CAD build for the part. Positions are in the model's coordinates, mm. A direction names the side the tool comes from. Coordinates: 2 decimals unless noted, no trailing zeros. Write each loop counter-clockwise with the first axis right and the second up, starting at its lowest first coordinate (ties: lowest second). Pieces come first, ordered by that corner, then holes.
```python
from build123d import *

# Parameters (mm, degrees)
BOX010_W               = 4
BOX010_H               = 10
BOX010_DEPTH           = 7
BOX010_PLACEMENT_ANGLE = 95
BOX009_W               = 4
BOX009_H               = 10
BOX009_DEPTH           = 7
BOX009_PLACEMENT_ANGLE = 45
BOX011_W               = 3.5
BOX011_H               = 10
BOX011_DEPTH           = 6.9
BOX008_W               = 3.5
BOX008_H               = 10
BOX008_DEPTH           = 6.9
CUT007_PLACEMENT_ANGLE = 180
BOX006_W               = 4
BOX006_H               = 10
BOX006_DEPTH           = 7
BOX006_PLACEMENT_ANGLE = 95
BOX005_W               = 4
BOX005_H               = 10
BOX005_DEPTH           = 7
BOX005_PLACEMENT_ANGLE = 45
BOX007_W               = 3.5
BOX007_H               = 10
BOX007_DEPTH           = 6.9
BOX004_W               = 3.5
BOX004_H               = 10
BOX004_DEPTH           = 6.9
BOX003_W               = 34
BOX003_H               = 34
BOX003_DEPTH           = 10
SKETCH002_W            = 40
SKETCH002_H            = 90
PAD001_DEPTH           = 2


with BuildPart() as cube010:
    # Box010 → Box010 (new body)
    with BuildSketch(Plane.XY):
        with Locations((2, 5)):
            Rectangle(BOX010_W, BOX010_H)
    extrude(amount=BOX010_DEPTH)


with BuildPart() as cube010_1:
    # Box010 placement: moved
    add(cube010.part.moved(Location((18.35, -13, 15.9))).rotate(Axis((18.35, -13, 15.9), (0, 1, 0)), BOX010_PLACEMENT_ANGLE))


with BuildPart() as fusion003:
    # Box009 → Box009 (new body)
    with BuildSketch(Plane.XY):
        with Locations((2, 5)):
            Rectangle(BOX009_W, BOX009_H)
    extrude(amount=BOX009_DEPTH)


with BuildPart() as fusion003_1:
    # Box009 placement: moved
    add(fusion003.part.moved(Location((16, -13, 7))).rotate(Axis((16, -13, 7), (0, 1, 0)), BOX009_PLACEMENT_ANGLE))

    # Fusion003: union Cube010
    add(cube010_1.part)


with BuildPart() as fusion004:
    # Box011 → Box011 (new body)
    with BuildSketch(Plane(origin=(18, -13, 12), x_dir=(1, 0, 0), z_dir=(0, 0, 1))):
        with Locations((1.75, 5)):
            Rectangle(BOX011_W, BOX011_H)
    extrude(amount=BOX011_DEPTH)

    # Fusion004: union Fusion003
    add(fusion003_1.part)


with BuildPart() as obj1:
    # Box008 → Box008 (new body)
    with BuildSketch(Plane(origin=(16.5, -13, 9.1), x_dir=(1, 0, 0), z_dir=(0, 0, 1))):
        with Locations((1.75, 5)):
            Rectangle(BOX008_W, BOX008_H)
    extrude(amount=BOX008_DEPTH)

    # Cut007: cut Fusion004
    add(fusion004.part, mode=Mode.SUBTRACT)


with BuildPart() as obj1_1:
    # Cut007 placement: moved
    add(obj1.part.moved(Location((0, -16, 0))).rotate(Axis((0, -16, 0), (0, 0, 1)), CUT007_PLACEMENT_ANGLE))


with BuildPart() as cube006:
    # Box006 → Box006 (new body)
    with BuildSketch(Plane.XY):
        with Locations((2, 5)):
            Rectangle(BOX006_W, BOX006_H)
    extrude(amount=BOX006_DEPTH)


with BuildPart() as cube006_1:
    # Box006 placement: moved
    add(cube006.part.moved(Location((18.35, -13, 15.9))).rotate(Axis((18.35, -13, 15.9), (0, 1, 0)), BOX006_PLACEMENT_ANGLE))


with BuildPart() as fusion001:
    # Box005 → Box005 (new body)
    with BuildSketch(Plane.XY):
        with Locations((2, 5)):
            Rectangle(BOX005_W, BOX005_H)
    extrude(amount=BOX005_DEPTH)


with BuildPart() as fusion001_1:
    # Box005 placement: moved
    add(fusion001.part.moved(Location((16, -13, 7))).rotate(Axis((16, -13, 7), (0, 1, 0)), BOX005_PLACEMENT_ANGLE))

    # Fusion001: union Cube006
    add(cube006_1.part)


with BuildPart() as fusion002:
    # Box007 → Box007 (new body)
    with BuildSketch(Plane(origin=(18, -13, 12), x_dir=(1, 0, 0), z_dir=(0, 0, 1))):
        with Locations((1.75, 5)):
            Rectangle(BOX007_W, BOX007_H)
    extrude(amount=BOX007_DEPTH)

    # Fusion002: union Fusion001
    add(fusion001_1.part)


with BuildPart() as obj2:
    # Box004 → Box004 (new body)
    with BuildSketch(Plane(origin=(16.5, -13, 9.1), x_dir=(1, 0, 0), z_dir=(0, 0, 1))):
        with Locations((1.75, 5)):
            Rectangle(BOX004_W, BOX004_H)
    extrude(amount=BOX004_DEPTH)

    # Cut006: cut Fusion002
    add(fusion002.part, mode=Mode.SUBTRACT)

    # Fusion005: union obj1
    add(obj1_1.part)


with BuildPart() as cube003:
    # Box003 → Box003 (new body)
    with BuildSketch(Plane(origin=(-17, 7, 10), x_dir=(1, 0, 0), z_dir=(0, 0, 1))):
        with Locations((17, 17)):
            Rectangle(BOX003_W, BOX003_H)
    extrude(amount=BOX003_DEPTH)


with BuildPart() as obj3:
    # Sketch002 → Pad001 (new body)
    with BuildSketch(Plane.XY.offset(16)):
        Rectangle(SKETCH002_W, SKETCH002_H)
    extrude(amount=PAD001_DEPTH)

    # Cut005: cut Cube003
    add(cube003.part, mode=Mode.SUBTRACT)

    # Fusion006: union obj2
    add(obj2.part)


solid = obj3.part
```
Item 1: Saw through at C-C, the plane z = 17. Write the cut outline in (x, y).
Item 2: Wall check: line 1 along Z through (x, y) = (11, 1); line 2 along X through (y, z) = (-4.5, 14); line 3 along Y through (x, z) = (12, 17). Give the ranges that are in metal, low to high.
Item 3: Two-plate mould, pull along X, no slides. Class faces 6 (the flat face through (-17, -8, 9.1)), 7 (the flat face through (0, 7, 17)), 8 (the flat face through (-18, -8, 14)): +X half, -X half, draft (parallel to the pull), parting line (faces both ways), or undercut.
Item 4: Saw through at A-A, the plane x = 1. Write the cut outline in (y, z), and give its area (3 significant figures).
Item 5: Flat gauge pins, fed straight in: pin 1 Ø2 at (x, y) = (8.5, -30.5) entering from -Z; pin 2 Ø3 at (x, z) = (18, 14) entering from -Y; pin 3 Ø1.5 at (x, z) = (3, 15) entering from -Y; pin 4 Ø4 at (x, z) = (-18, 12) entering from +Y. Where does each tip first touch, or does it go through?
Item 6: Which spindle directions (+Z, -Z, +X, -X, +Y, -Y) get a long thin tool onto all of the face, cutting with end or side? Do faces 1 (the flat face through (-18.99, -7.93, 11.83)), 2 (the flat face through (18.99, -8.07, 11.83)), 3 (the flat face through (-17.8, -3, 11.7)), 4 (the flat face through (-17, 24, 17)), 5 (the flat face through (-16.5, -8, 13)). Say none if no direction does.
Item 7: Saw through at B-B, the plane z = 13. Write the cut outline in (x, y), and give its area (3 significant figures).
Working result:
1. outline: (-20, -45) - (20, -45) - (20, 45) - (-20, 45) - close; hole (-17, 7) - (17, 7) - (17, 41) - (-17, 41) - close
2. line 1: z = 16 to 18
2. line 2: x = -18 to -16.5, 16.5 to 18
2. line 3: y = -45 to 7, 41 to 45
3. face 6: draft
3. face 7: undercut
3. face 8: -X half
4. outline: (-45, 16) - (7, 16) - (7, 18) - (-45, 18) - close; (41, 16) - (45, 16) - (45, 18) - (41, 18) - close
4. area: 112 mm2
5. pin 1: stops at z = 16
5. pin 2: stops at y = -13
5. pin 3: passes through
5. pin 4: stops at y = -3
6. face 1: -X, +Y, -Y
6. face 2: +X, +Y, -Y
6. face 3: -Z, +X, -X, +Y
6. face 4: +Z, -Z
6. face 5: -Z, +Y, -Y
7. outline: (-18, -13) - (-16.5, -13) - (-16.5, -3) - (-18, -3) - close; (16.5, -13) - (18, -13) - (18, -3) - (16.5, -3) - close
7. area: 30.0 mm2
